Source: CAD feature listing. Evaluate the final solid. Frame: model axes, mm. A direction names the side the tool comes from. Coordinates: 2 decimals unless noted, no trailing zeros. Write each loop counter-clockwise with the first axis right and the second up, starting at its lowest first coordinate (ties: lowest second). Pieces come first, ordered by that corner, then holes. Notation, with made-up numbers: (-5, 41.5) - (21, 41.5) arc R22 cw to (21, 49.5) - close; hole circle Ø8 at (55.5, 2). An arc over 180 degrees is marked (long way). One line per question, with ' | ' between items. Start each with the question number.
Q1. Access query for faces 4 (the face through (9, 1, 13)), 5 (the face through (33, 34, 17)), 6 (the face through (22.54, -3.07, 10.04)). Directions: +Z, -Z, +X, -X, +Y, -Y. A direction counts if a zero-diameter tool reaches every point of the face in a straight line with its end or side. Return the directions, or none.
Q2. Draft query along Y for faces 1 (the face through (-41, 19, 20)), 2 (the face through (47.69, 15.02, 18.48)), 3 (the face through (-4.618, 1.917, 10.042)). Return one class per face: +Y half, -Y half, draft (parallel to the pull), parting line (faces both ways), or undercut.
Q3. Cut plane B-B, the plane z = 9.5. Return loops of the section in (x, y), plus the area to 3 significant figures.
Q4. Contact query for flat-ended pins moving along their axis: P1, Ø1.8, axis at x = 0, y = 0, coming from the -Z side; P2, Ø1.5, axis at y = -9, z = 17.5, coming from the +X side; P3, Ø5, axis at x = 38, z = 3.5, coming from the +Y side; P4, Ø2, axis at y = 33.5, z = 9, coming from the -X side. Output: stop coordinate, or through.
Q5. Cut plane C-C, the plane x = -22.5. Return loops of the section in (y, z), plus the area to 3 significant figures.
Q6. Cut plane A-A, the plane y = 13. Give the number of separate pieces and of enclosed holes in the cut face, plus the area to 3 significant figures.
Q7. Line query: line 1 (Y direction, x = 0, z = 11.4); line 2 (Y direction, x = -28, z = 10.5); line 3 (Y direction, x = 0, z = 3.5). Output: solid intervals per line, ascending.
Q8. Cut plane D-D, the plane y = -41.5. Return loops of the section in (x, z).
```python
from build123d import *

# Parameters (mm, degrees)
ESQUISSE2_R             = 50
BOSS_EXTRU_1_DEPTH      = 20
ESQUISSE3_R             = 45
ENL_V_MAT_EXTRU_1_DEPTH = 7
ESQUISSE4_R             = 45
ENL_V_MAT_EXTRU_2_DEPTH = 7
ENL_V_MAT_EXTRU_3_DEPTH = 14
ESQUISSE7_W             = 14
ESQUISSE7_H             = 4.126499196
ESQUISSE8_R             = 1.5
ENL_V_MAT_EXTRU_4_DEPTH = 21


with BuildPart() as part:
    # Esquisse2 → Boss.-Extru.1 (new body)
    with BuildSketch(Plane.XY):
        Circle(ESQUISSE2_R)
    extrude(amount=BOSS_EXTRU_1_DEPTH)

    # Esquisse3 → Enlèv. mat.-Extru.1 (cut)
    with BuildSketch(Plane.XY):
        Circle(ESQUISSE3_R)
    extrude(amount=ENL_V_MAT_EXTRU_1_DEPTH, mode=Mode.SUBTRACT)

    # Esquisse4 → Enlèv. mat.-Extru.2 (cut)
    with BuildSketch(Plane.XY.offset(20)):
        Circle(ESQUISSE4_R)
    extrude(amount=-ENL_V_MAT_EXTRU_2_DEPTH, mode=Mode.SUBTRACT)

    # Esquisse6 → Enlèv. mat.-Extru.3 (cut, through all)
    with BuildSketch(Plane.XY.offset(13)):
        with BuildLine():
            ThreePointArc((3.061476111, 3.953146092), (3.980308338, 3.026077582), (4.627889131, 1.892786885))
            Line((4.627889131, 1.892786885), (37.023113047, 15.142295082))
            ThreePointArc((37.023113047, 15.142295082), (31.842466708, 24.208620654), (24.491808885, 31.625168736))
            Line((24.491808885, 31.625168736), (3.061476111, 3.953146092))
        make_face()
        with BuildLine():
            ThreePointArc((-1.892786885, 4.627889131), (-0.63050589, 4.960086927), (0.674743039, 4.954262996))
            Line((0.674743039, 4.954262996), (5.397944311, 39.634103966))
            ThreePointArc((5.397944311, 39.634103966), (-5.044047123, 39.680695415), (-15.142295082, 37.023113047))
            Line((-15.142295082, 37.023113047), (-1.892786885, 4.627889131))
        make_face()
        with BuildLine():
            ThreePointArc((-4.954262996, 0.674743039), (-4.610814229, 1.934009345), (-3.953146092, 3.061476111))
            Line((-3.953146092, 3.061476111), (-31.625168736, 24.491808885))
            ThreePointArc((-31.625168736, 24.491808885), (-36.886513831, 15.472074761), (-39.634103966, 5.397944311))
            Line((-39.634103966, 5.397944311), (-4.954262996, 0.674743039))
        make_face()
        with BuildLine():
            Line((-24.491808885, -31.625168736), (-3.061476111, -3.953146092))
            ThreePointArc((-3.061476111, -3.953146092), (-3.980308338, -3.026077582), (-4.627889131, -1.892786885))
            Line((-4.627889131, -1.892786885), (-37.023113047, -15.142295082))
            ThreePointArc((-37.023113047, -15.142295082), (-31.842466708, -24.208620654), (-24.491808885, -31.625168736))
        make_face()
        with BuildLine():
            Line((15.142295082, -37.023113047), (1.892786885, -4.627889131))
            ThreePointArc((1.892786885, -4.627889131), (0.63050589, -4.960086927), (-0.674743039, -4.954262996))
            Line((-0.674743039, -4.954262996), (-5.397944311, -39.634103966))
            ThreePointArc((-5.397944311, -39.634103966), (5.044047123, -39.680695415), (15.142295082, -37.023113047))
        make_face()
        with BuildLine():
            Line((39.634103966, -5.397944311), (4.954262996, -0.674743039))
            ThreePointArc((4.954262996, -0.674743039), (4.610814229, -1.934009345), (3.953146092, -3.061476111))
            Line((3.953146092, -3.061476111), (31.625168736, -24.491808885))
            ThreePointArc((31.625168736, -24.491808885), (36.886513831, -15.472074761), (39.634103966, -5.397944311))
        make_face()
    extrude(amount=-ENL_V_MAT_EXTRU_3_DEPTH, mode=Mode.SUBTRACT)

    # Esquisse7 → Enlèvement de matière-Révolution1 (revolve, cut)
    with BuildSketch(Plane(origin=(0, 0, 0), x_dir=(0, 0, -1), z_dir=(1, 0, 0))):
        with Locations((-10, 49.063249598)):
            Rectangle(ESQUISSE7_W, ESQUISSE7_H)
    revolve(axis=Axis((0, 0, 0), (0, 0, 1)), mode=Mode.SUBTRACT)

    # Esquisse8 → Enlèv. mat.-Extru.4 (cut, through all)
    with BuildSketch(Plane.XY):
        Circle(ESQUISSE8_R)
    extrude(amount=ENL_V_MAT_EXTRU_4_DEPTH, mode=Mode.SUBTRACT)


solid = part.part
```
Reply:
1) face 4: +Z | face 5: none | face 6: +Z, -Z
2) face 1: draft | face 2: parting line | face 3: undercut
3) outline: circle Ø94 at (0, 0); hole (-39.63, 5.4) - (-4.95, 0.67) arc R5 cw to (-3.95, 3.06) - (-31.63, 24.49) arc R40 ccw to start; hole (-37.02, -15.14) arc R40 ccw to (-24.49, -31.63) - (-3.06, -3.95) arc R5 cw to (-4.63, -1.89) - close; hole (-15.14, 37.02) - (-1.89, 4.63) arc R5 cw to (0.67, 4.95) - (5.4, 39.63) arc R40 ccw to start; hole (-5.4, -39.63) arc R40 ccw to (15.14, -37.02) - (1.89, -4.63) arc R5 cw to (-0.67, -4.95) - close; hole circle Ø3 at (0, 0); hole (3.06, 3.95) arc R5 cw to (4.63, 1.89) - (37.02, 15.14) arc R40 ccw to (24.49, 31.63) - close; hole (3.95, -3.06) - (31.63, -24.49) arc R40 ccw to (39.63, -5.4) - (4.95, -0.67) arc R5 cw to start | area: 4,460 mm^2
4) P1: passes through | P2: stops at x = 49.31 | P3: stops at y = 35.16 | P4: stops at x = -33.95
5) outline: (-44.65, 0) - (-38.97, 0) - (-38.97, 7) - (-29.05, 7) - (-29.05, 13) - (-38.97, 13) - (-38.97, 20) - (-44.65, 20) - (-44.65, 17) - (-41.26, 17) - (-41.26, 3) - (-44.65, 3) - close; (-9.2, 7) - (3.06, 7) - (3.06, 13) - (-9.2, 13) - close; (17.42, 7) - (38.97, 7) - (38.97, 0) - (44.65, 0) - (44.65, 3) - (41.26, 3) - (41.26, 17) - (44.65, 17) - (44.65, 20) - (38.97, 20) - (38.97, 13) - (17.42, 13) - close | area: 395 mm^2
6) separate pieces: 4 | enclosed holes: 0 | area: 339 mm^2
7) line 1: y = -47 to -40, -5 to -1.5, 1.5 to 5, 40 to 47 | line 2: y = -37.75 to -28.57, -11.45 to 3.81, 21.68 to 37.75 | line 3: y = -47 to -45, 45 to 47
8) outline: (-27.89, 0) - (-17.4, 0) - (-17.4, 7) - (17.4, 7) - (17.4, 0) - (27.89, 0) - (27.89, 3) - (22.06, 3) - (22.06, 17) - (27.89, 17) - (27.89, 20) - (17.4, 20) - (17.4, 13) - (-17.4, 13) - (-17.4, 20) - (-27.89, 20) - (-27.89, 17) - (-22.06, 17) - (-22.06, 3) - (-27.89, 3) - close
